```python
from build123d import *

# Parameters (mm, degrees)
BOSS_EXTRUDE1_DEPTH = 12.7
CHAMFER2_SIZE       = 12.7
CHAMFER2_SIZE2      = 6.35
CHAMFER3_SIZE       = 31.75
CHAMFER3_SIZE2      = 9.525
SKETCH2_R           = 7.9375
CUT_EXTRUDE1_DEPTH  = 13.7


with BuildPart() as part:
    # Sketch1 → Boss-Extrude1 (new body)
    with BuildSketch(Plane(origin=(0, 0, 0), x_dir=(1, 0, 0), z_dir=(0, 1, 0))):
        with BuildLine():
            Line((0, 31.75), (120.65, 31.75))
            Line((120.65, 31.75), (120.65, -31.75))
            Line((120.65, -31.75), (0, -31.75))
            ThreePointArc((0, -31.75), (-31.75, 0), (0, 31.75))
        make_face()
    extrude(amount=BOSS_EXTRUDE1_DEPTH)

    # Chamfer2
    chamfer2_edges = [part.edges().sort_by_distance(p)[0] for p in [
        (60.325, 12.7, 31.75),
        (-31.75, 12.7, 0),
        (60.325, 12.7, -31.75),
    ]]
    chamfer2_side = [part.faces().sort_by_distance(p)[0] for p in [
        (47.684335989, 12.7, 0),
    ]]
    chamfer(chamfer2_edges, length=CHAMFER2_SIZE, length2=CHAMFER2_SIZE2, reference=chamfer2_side[0])

    # Chamfer3
    chamfer3_edges = [part.edges().sort_by_distance(p)[0] for p in [
        (120.65, 12.7, 0),
    ]]
    chamfer3_side = [part.faces().sort_by_distance(p)[0] for p in [
        (52.777427201, 12.7, 0),
    ]]
    chamfer(chamfer3_edges, length=CHAMFER3_SIZE, length2=CHAMFER3_SIZE2, reference=chamfer3_side[0])

    # Sketch2 → Cut-Extrude1 (cut, through all)
    with BuildSketch(Plane(origin=(0, 12.7, 0), x_dir=(1, 0, 0), z_dir=(0, 1, 0))):
        Circle(SKETCH2_R)
        with Locations((25.4, 0)):
            Circle(SKETCH2_R)
        with Locations((50.8, 0)):
            Circle(SKETCH2_R)
        with Locations((76.2, 0)):
            Circle(SKETCH2_R)
    extrude(amount=-CUT_EXTRUDE1_DEPTH, mode=Mode.SUBTRACT)


solid = part.part
```
Can you work these out from the model? Positions are in its coordinate system, mm. Give positions to 0.01 mm unless a question says otherwise; leave off trailing zeros. Loops run counter-clockwise (first coordinate to the right, second up) from the corner with the lowest first, then second, coordinate; pieces in that order, holes last. Notation, with made-up numbers: M 58.25,-27 L 97.25,-27 A15 ccw 97.25,-17 Z; hole C 21.5,63 d7. An arc over 180 degrees is marked long. One line per item, written item: value.
(1) Will these pins go through, and if not, where does the flat tip stop? pin 1 (12.5 mm diameter, centred on x = 76.2, z = 0, fed in from +Y); pin 2 (6 mm diameter, centred on y = 8, z = -24, fed in from -X).
Returned:
pin 1: through
pin 2: x = -23.37
(2) Suppose I cut it at B-B on z = 0. Count the separate pieces of the cut face and the enclosed holes in it, plus the area to 4 significant figures.
Returned:
separate pieces: 5
enclosed holes: 0
area: 937.5 mm^2
(3) We'd pull the mould along Z, two halves only. Please class faces 1 (the face through (17.47, 6.44, -0.35)), 2 (the face through (61, 3, 31.75)), 3 (the face through (36, 12.7, 0)): released by +Z, released by -Z, zero draft, split by the parting line, or undercut.
Returned:
face 1: undercut
face 2: released by +Z
face 3: zero draft
(4) I need wall thicknesses on line 1 (Z direction, x = 25.4, y = 5.5); line 2 (X direction, y = 3, z = 0). Which ranges of each line are inside material? Lowest first, please.
Returned:
line 1: -31.75 to -7.94, 7.94 to 31.75
line 2: -31.75 to -7.94, 7.94 to 17.46, 33.34 to 42.86, 58.74 to 68.26, 84.14 to 120.65
(5) Suppose I cut it at A-A on x = 76.2. List the corners of the cut face in (y, z) for me.
Returned:
outline: M 0,-31.75 L 6.35,-31.75 L 12.7,-19.05 L 12.7,-7.94 L 0,-7.94 Z; M 0,7.94 L 12.7,7.94 L 12.7,19.05 L 6.35,31.75 L 0,31.75 Z
(6) Suppose I cut it at D-D on x = 27. List the corners of the cut face in (y, z) for me.
Returned:
outline: M 0,-31.75 L 6.35,-31.75 L 12.7,-19.05 L 12.7,-7.77 L 0,-7.77 Z; M 0,7.77 L 12.7,7.77 L 12.7,19.05 L 6.35,31.75 L 0,31.75 Z
